from build123d import *

# Parameters (mm, degrees)
F0_W       = 440
F0_H       = 123
F1_DEPTH   = 364
F2_R       = 40
F3_DEPTH   = 25
F4_W       = 209.3812078238
F4_H       = 68.7625966966
F5_DEPTH   = 50
F6_SIZE2   = 2.99999
F6_SIZE    = 49.99999
F6_2_SIZE2 = 2.99999
F6_2_SIZE  = 49.99999
F7_R       = 5


# Not quite as in the source:
# - a fillet or chamfer is up to 0.001 mm smaller than in the source, because OpenCascade refuses the exact size


with BuildPart() as f1:
    # F0 (on Front) → F1 (new body)
    with BuildSketch(Plane.XZ):
        Rectangle(F0_W, F0_H)
    extrude(amount=F1_DEPTH)

    # F2 (on face) → F3 (join)
    with BuildSketch(Plane(origin=(0, 0, 0), x_dir=(-1, 0, 0), z_dir=(0, 1, 0))):
        with Locations((-160, 0)):
            Circle(F2_R)
        with Locations((160, 0)):
            Circle(F2_R)
    extrude(amount=F3_DEPTH)

    # F4 (on face) → F5 (join)
    with BuildSketch(Plane.XZ.offset(364)):
        with Locations((91.689683497, -0.3388542682)):
            Rectangle(F4_W, F4_H)
    extrude(amount=F5_DEPTH)

    # F6 (size 50 and 3 in the source; OpenCascade refuses exactly that, so slightly less here)
    f6_edges = [f1.edges().sort_by_distance(p)[0] for p in [
        (91.689683, -414, 34.042444),
    ]]
    f6_side = f1.faces().sort_by_distance((91.689683, -389, 34.042444))[0]
    chamfer(f6_edges, length=F6_SIZE, length2=F6_SIZE2, reference=f6_side)

    # F6#2 (size 50 and 3 in the source; OpenCascade refuses exactly that, so slightly less here)
    f6_2_edges = [f1.edges().sort_by_distance(p)[0] for p in [
        (91.689683, -414, -34.720153),
    ]]
    f6_2_side = f1.faces().sort_by_distance((91.689683, -389, -34.720153))[0]
    chamfer(f6_2_edges, length=F6_2_SIZE, length2=F6_2_SIZE2, reference=f6_2_side)

    # F7
    f7_edges = [f1.edges().sort_by_distance(p)[0] for p in [
        (91.689683, -414, 31.042454),
        (91.689683, -414, -31.720163),
    ]]
    fillet(f7_edges, radius=F7_R)


solid = f1.part
Build history of the part. All positions in model axes, mm. A direction names the side the tool comes from. Round coordinates to 2 decimals unless told otherwise and drop trailing zeros. Write each loop counter-clockwise with the first axis right and the second up, starting at its lowest first coordinate (ties: lowest second). Pieces come first, ordered by that corner, then holes. Notation, with made-up numbers: (-15, 67) -> (42, 67) arc R19 ccw to (42, 74) -> close; hole circle Ø4 at (24.25, 67.25). An arc over 180 degrees is marked (long way). Use one line per item in the form item = value.
Q1. Tool access for faces 1 (the flat face through (90.224, -386.967, 32.664)), 2 (the flat face through (-13.001, -389, -1)), 3 (the flat face through (-3, -179, -61.5)), 4 (the cylindrical face through (199.96, 12.32, 1.76)), 5 (the flat face through (196.38, -389, -1)): list every direction of +Z, -Z, +X, -X, +Y, -Y with a clear straight run to the whole face (end or side of a thin tool).
Conclusion:
face_1 = +Z, +X, -X, -Y
face_2 = +Z, -Z, -X, -Y
face_3 = -Z, +X, -X, +Y, -Y
face_4 = +Y
face_5 = +Z, -Z, +X, -Y
Q2. Drill centre lines: L1, parallel to Y at x = -139.5, z = 56; L2, parallel to Y at x = 85, z = -12; L3, parallel to X at y = -375.5, z = 2. Where is each one in solid material? Low to high.
Conclusion:
L1 = -364 to 0
L2 = -414 to 0
L3 = -13 to 196.38
Q3. Drop flat-ended pins along their axis: P1, Ø6, axis at x = -69, z = -23.5, coming from the +Y side; P2, Ø1, axis at x = 112, y = -367.5, coming from the -Z side; P3, Ø8, axis at x = -95.5, z = 34.5, coming from the -Y side. Give the stop position or say it passes through.
Conclusion:
P1 = 0
P2 = -34.54
P3 = -364
Q4. Band-saw the part on A-A, the plane x = -160. Write the cut outline in (y, z).
Conclusion:
outline = (-364, -61.5) -> (0, -61.5) -> (0, -40) -> (25, -40) -> (25, 40) -> (0, 40) -> (0, 61.5) -> (-364, 61.5) -> close
Q5. Band-saw the part on B-B, the plane z = 0. Write the cut outline in (x, y), then the cut area to 3 significant figures.
Conclusion:
outline = (-220, -364) -> (-13, -364) -> (-13, -414) -> (196.38, -414) -> (196.38, -364) -> (220, -364) -> (220, 0) -> (200, 0) -> (200, 25) -> (120, 25) -> (120, 0) -> (-120, 0) -> (-120, 25) -> (-200, 25) -> (-200, 0) -> (-220, 0) -> close
area = 175,000 mm²
Q6. Band-saw the part on D-D, the plane z = 46. Write the cut outline in (x, y), then the cut area to 3 significant figures.
Conclusion:
outline = (-220, -364) -> (220, -364) -> (220, 0) -> (-220, 0) -> close
area = 160,000 mm²
Q7. Two-plate mould, pull along X, no slides. Class faces 6 (the flat face through (-220, -179, -1)), 7 (the flat face through (-3, -179, 61.5)), 8 (the flat face through (-3, 0, 1)): released by +X, released by -X, zero draft, split by the parting line, or undercut.
Conclusion:
face_6 = released by -X
face_7 = zero draft
face_8 = undercut
